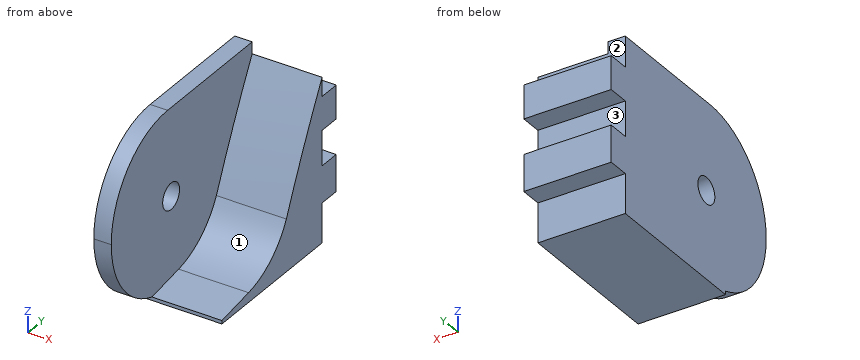
from build123d import *

# Parameters (mm, degrees)
DODANIE_WYCI_GNI_CIE1_DEPTH = 40
ZAOKR_GLENIE1_R             = 20
DODANIE_WYCI_GNI_CIE2_DEPTH = 20
SZKIC6_R                    = 3
WYTNIJ_WYCI_GNI_CIE1_DEPTH  = 10
WYTNIJ_WYCI_GNI_CIE2_DEPTH  = 71.887234394


with BuildPart() as part:
    # Szkic1 → Dodanie-wyciągnięcie1 (new body)
    with BuildSketch(Plane.XY):
        Polygon((0, 0), (-4, 0), (-4, 55), (16, 55), (16, 51.5), (0, 51.5), align=None)
    extrude(amount=DODANIE_WYCI_GNI_CIE1_DEPTH)

    # Zaokrąglenie1
    zaokr_glenie1_edges = [part.edges().sort_by_distance(p)[0] for p in [
        (-2, 0, 0),
        (-2, 0, 40),
    ]]
    fillet(zaokr_glenie1_edges, radius=ZAOKR_GLENIE1_R - 0.0001)  # a hair under: the kernel refuses the full size

    # Szkic5 → Dodanie-wyciągnięcie2 (add)
    with BuildSketch(Plane.ZY.offset(4)):
        with BuildLine():
            ThreePointArc((0.786266298, 14.447303609), (0.197542147, 17.19595596), (0, 20))
            Line((0, 20), (0, 14.447303609))
            Line((0, 14.447303609), (0.786266298, 14.447303609))
        make_face()
        with BuildLine():
            Line((40, 51.5), (0, 51.5))
            Line((0, 51.5), (0, 20))
            ThreePointArc((0, 20), (0.197542147, 17.19595596), (0.786266298, 14.447303609))
            Line((0.786266298, 14.447303609), (2.19744111, 23.896337815))
            ThreePointArc((2.19744111, 23.896337815), (5.410467594, 31.78015679), (11.887142793, 37.30562683))
            Line((11.887142793, 37.30562683), (40, 51.5))
        make_face()
        with BuildLine():
            ThreePointArc((40, 51.5), (26.114639544, 44.064002088), (11.887142793, 37.30562683))
            Line((11.887142793, 37.30562683), (40, 51.5))
        make_face()
    extrude(amount=-DODANIE_WYCI_GNI_CIE2_DEPTH)

    # Szkic6 → Wytnij-wyciągnięcie1 (cut)
    with BuildSketch(Plane.ZY.offset(4)):
        with Locations((20, 21.237598079)):
            Circle(SZKIC6_R)
    extrude(amount=-WYTNIJ_WYCI_GNI_CIE1_DEPTH, mode=Mode.SUBTRACT)

    # Szkic8 → Wytnij-wyciągnięcie2 (cut, through all)
    with BuildSketch(Plane.ZY.offset(4)):
        Polygon((0, 50), (9, 50), (9, 55), (17.366037593, 55), (17.366037593, 50), (25.366037593, 50), (25.366037593, 55), (33, 55), (33, 50), (40, 50), (40, 57.074314744), (0, 57.074314744), align=None)
    extrude(amount=-WYTNIJ_WYCI_GNI_CIE2_DEPTH, mode=Mode.SUBTRACT)


solid = part.part
Read the model definition and answer for the solid it produces. Units are mm, in the model's axes. Face numbers are marked on the shaded views. A direction names the side the tool comes from. Give positions to 0.01 mm unless a question says otherwise; leave off trailing zeros. Loops run counter-clockwise (first coordinate to the right, second up) from the corner with the lowest first, then second, coordinate; pieces in that order, holes last. Notation, with made-up numbers: (-30, -37) -> (-13, -37) arc R9 ccw to (-13, -22) -> close; hole circle Ø4 at (63.5, -5). An arc over 180 degrees is marked (long way). Use a Markdown table: item, result.
Q1. Find the intervals of material crossed by line 1 along Y through (x, z) = (-2.2, 20); line 2 along Z through (x, y) = (8.5, 51.5); line 3 along X through (y, z) = (49, 38), in increasing order.
Solved:
| item | result |
|---|---|
| line 1 | y = 0 to 18.24, 24.24 to 50 |
| line 2 | z = 9 to 17.37, 25.37 to 33 |
| line 3 | x = -4 to 0 |
Q2. Section D-D, the plane z = 30.5 is taken. Determine the outline of the cut face in (x, y).
Solved:
| item | result |
|---|---|
| outline | (-4, 2.98) -> (0, 2.98) -> (0, 46.32) -> (16, 46.32) -> (16, 55) -> (-4, 55) -> close |
Q3. A tool of negligible diameter and unlimited length cuts with its end or side. For the marked faces 1, 2 and 3, from which of +Z, -Z, +X, -X, +Y, -Y can it reach the whole face along a straight path? Write none if from no direction.
Solved:
| item | result |
|---|---|
| face 1 | +Z, +X, -Y |
| face 2 | +Z, +X, -X, +Y |
| face 3 | +X, -X, +Y |
Q4. Section A-A, the plane z = 21 is taken. Determine the outline of the cut face in (x, y), then the cut area to 3 significant figures.
Solved:
| item | result |
|---|---|
| outline | (-4, 0.03) -> (0, 0.03) -> (0, 18.41) -> (-4, 18.41) -> close; (-4, 24.07) -> (0, 24.07) -> (0, 41.54) -> (16, 41.54) -> (16, 50) -> (-4, 50) -> close |
| area | 313 mm^2 |
Q5. Each of these flat-tipped pins is pushed along its axis until it touches: pin 1 (9.5 mm diameter, centred on y = 21.24, z = 20, fed in from +X); pin 2 (3 mm diameter, centred on x = 9, y = 23, fed in from +Z); pin 3 (1.5 mm diameter, centred on x = 2, y = 53, fed in from -Z); pin 4 (1 mm diameter, centred on x = 4, y = 31.5, fed in from -Z). Where does it stop, or does it pass through?
Solved:
| item | result |
|---|---|
| pin 1 | stops at x = 0 |
| pin 2 | stops at z = 2.3 |
| pin 3 | stops at z = 9 |
| pin 4 | stops at z = 0 |
Q6. Section B-B, the plane x = 11.5 is taken. Determine the outline of the cut face in (y, z), then the cut area to 3 significant figures.
Solved:
| item | result |
|---|---|
| outline | (14.45, 0) -> (50, 0) -> (50, 9) -> (55, 9) -> (55, 17.37) -> (50, 17.37) -> (50, 25.37) -> (55, 25.37) -> (55, 33) -> (50, 33) -> (50, 37.33) arc R326.83 ccw to (37.31, 11.89) arc R18 cw to (23.9, 2.2) -> (14.45, 0.79) -> close |
| area | 484 mm^2 |
